Model file for the job. Use its own axes, mm. Face numbers are marked on the shaded views. A direction names the side the tool comes from. Coordinates: 2 decimals unless noted, no trailing zeros. Order: outer loops, then holes, each group sorted by start corner. A loop starts at its lowest first (then second) coordinate and runs counter-clockwise, first axis right, second up.
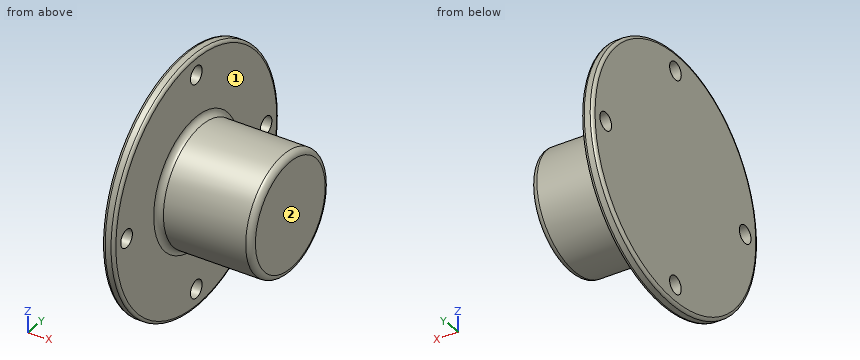
from build123d import *

# Parameters (mm, degrees)
CUT_EXTRUDE1_REACH = 36.046
SKETCH3_R          = 1.5
CIRPATTERN1_COUNT  = 4
FILLET1_R          = 0.5
FILLET2_R          = 1


with BuildPart() as part:
    # Sketch2 → Revolve1 (revolve)
    with BuildSketch(Plane.XY):
        Polygon((0, 0), (0, 21.25), (2, 21.25), (2, 10), (18, 10), (18, 0), align=None)
    revolve(axis=Axis((18, 0, 0), (-1, 0, 0)))

    # Sketch3 → Cut-Extrude1 (cut, up to next)
    with BuildSketch(Plane(origin=(2, 0, 0), x_dir=(0, 0, -1), z_dir=(1, 0, 0)), mode=Mode.PRIVATE) as cut_extrude1_sk1:
        with Locations(Location((0, 18, 0), (0, 0, 90))):
            Circle(SKETCH3_R)
    cut_extrude1_tool1 = extrude(cut_extrude1_sk1.sketch, amount=-CUT_EXTRUDE1_REACH, mode=Mode.PRIVATE) & part.part
    cut_extrude1 = cut_extrude1_tool1.solids().sort_by_distance((2, 18, 0))[0]
    add(cut_extrude1, mode=Mode.SUBTRACT)

    # CirPattern1: Cut-Extrude1 ×4 about axis
    cirpattern1_axis = Axis((0, 0, 0), (1, 0, 0))
    for i in range(1, CIRPATTERN1_COUNT):
        add(cut_extrude1.rotate(cirpattern1_axis, i * 360 / CIRPATTERN1_COUNT), mode=Mode.SUBTRACT)

    # Fillet1
    fillet1_edges = [part.edges().sort_by_distance(p)[0] for p in [
        (2, -21.25, 0),
        (0, -21.25, 0),
    ]]
    fillet(fillet1_edges, radius=FILLET1_R)

    # Fillet2
    fillet2_edges = [part.edges().sort_by_distance(p)[0] for p in [
        (18, -10, 0),
        (2, -10, 0),
    ]]
    fillet(fillet2_edges, radius=FILLET2_R)


solid = part.part
Q1. Cut at A-A, the plane y = 0. List the corners of the cut face in (x, z), plus the area to 3 significant figures.
Established:
outline: (0, -20.75) arc R0.5 ccw to (0.5, -21.25) - (1.5, -21.25) arc R0.5 ccw to (2, -20.75) - (2, -19.5) - (0, -19.5) - close; (0, -16.5) - (2, -16.5) - (2, -11) arc R1 cw to (3, -10) - (17, -10) arc R1 ccw to (18, -9) - (18, 9) arc R1 ccw to (17, 10) - (3, 10) arc R1 cw to (2, 11) - (2, 16.5) - (0, 16.5) - close; (0, 19.5) - (2, 19.5) - (2, 20.75) arc R0.5 ccw to (1.5, 21.25) - (0.5, 21.25) arc R0.5 ccw to (0, 20.75) - close
area: 393 mm2
Q2. Which spindle directions (+Z, -Z, +X, -X, +Y, -Y) get a long thin tool onto all of the face, cutting with end or side? Do the marked faces 1 and 2. Say none if no direction does.
Established:
face 1: +X
face 2: +Z, -Z, +X, +Y, -Y
Q3. Probe line 1 (X direction, y = -11, z = 3); line 2 (Z direction, x = 1.6, y = -18); line 3 (Y direction, x = 10, z = 0.5). List the from-to ranges inside material, lowest first.
Established:
line 1: x = 0 to 2
line 2: z = -11.28 to -1.5, 1.5 to 11.28
line 3: y = -9.99 to 9.99
Q4. Drop flat-ended pins along their axis: P1, Ø4, axis at y = 18, z = 0, coming from the +X side; P2, Ø1, axis at x = 6.5, z = 0, coming from the -Y side; P3, Ø2, axis at x = 2, y = 4.5, coming from the +Z side; P4, Ø1.8, axis at y = 0, z = -18, coming from the -X side. Give the stop position or say it passes through.
Established:
P1: stops at x = 2
P2: stops at y = -10
P3: stops at z = 20.94
P4: passes through
Q5. Cut at C-C, the plane x = 8. List the corners of the cut face in (y, z).
Established:
outline: circle Ø20 at (0, 0)
